from build123d import *

# Parameters (mm, degrees)
SKETCH1_W           = 33.746
SKETCH1_H           = 13.93
SKETCH1_W_2         = 32.946
SKETCH1_H_2         = 13.13
BOSS_EXTRUDE1_DEPTH = 11.37
CUT_EXTRUDE1_DEPTH  = 25.658060122
BOSS_EXTRUDE2_DEPTH = 5
BOSS_EXTRUDE3_DEPTH = 5


with BuildPart() as part:
    # Sketch1 → Boss-Extrude1 (new, symmetric)
    with BuildSketch(Plane.XY):
        Rectangle(SKETCH1_W, SKETCH1_H)
        Rectangle(SKETCH1_W_2, SKETCH1_H_2, mode=Mode.SUBTRACT)
    extrude(amount=BOSS_EXTRUDE1_DEPTH, both=True)

    # Sketch3 → Cut-Extrude1 (cut, through all)
    with BuildSketch(Plane(origin=(0, 6.965, 0), x_dir=(1, 0, 0), z_dir=(0, 1, 0))):
        with BuildLine():
            ThreePointArc((0, 11.37), (8.54007907, 10.702927857), (16.873, 8.717892708))
            Line((16.873, 8.717892708), (16.873, 11.37))
            Line((16.873, 11.37), (0, 11.37))
        make_face()
        with BuildLine():
            Line((-16.873, 11.37), (-16.873, 8.717892708))
            ThreePointArc((-16.873, 8.717892708), (-8.54007907, 10.702927857), (0, 11.37))
            Line((0, 11.37), (-16.873, 11.37))
        make_face()
        with BuildLine():
            ThreePointArc((16.873, -11.37), (0, -7.1709728), (-16.873, -11.37))
            Line((-16.873, -11.37), (16.873, -11.37))
        make_face()
    extrude(amount=-CUT_EXTRUDE1_DEPTH, mode=Mode.SUBTRACT)

    # Sketch4 → Boss-Extrude2 (add)
    with BuildSketch(Plane(origin=(0, 6.965, 0), x_dir=(1, 0, 0), z_dir=(0, 1, 0))):
        with BuildLine():
            Line((-16.873, -11.37), (-16.873, -10.37))
            ThreePointArc((-16.873, -10.37), (0, -6.1709728), (16.873, -10.37))
            Line((16.873, -10.37), (16.873, -11.37))
            ThreePointArc((16.873, -11.37), (0, -7.1709728), (-16.873, -11.37))
        make_face()
        with BuildLine():
            Line((-16.873, 8.717892708), (-16.873, 7.717892708))
            ThreePointArc((-16.873, 7.717892708), (0, 10.37), (16.873, 7.717892708))
            Line((16.873, 7.717892708), (16.873, 8.717892708))
            ThreePointArc((16.873, 8.717892708), (0, 11.37), (-16.873, 8.717892708))
        make_face()
    extrude(amount=BOSS_EXTRUDE2_DEPTH)

    # Sketch5 → Boss-Extrude3 (add)
    with BuildSketch(Plane.XZ.offset(6.965)):
        with BuildLine():
            Line((-16.873, 11.37), (-16.873, 10.37))
            ThreePointArc((-16.873, 10.37), (0, 6.1709728), (16.873, 10.37))
            Line((16.873, 10.37), (16.873, 11.37))
            ThreePointArc((16.873, 11.37), (0, 7.1709728), (-16.873, 11.37))
        make_face()
        with BuildLine():
            Line((-16.873, -8.717892708), (-16.873, -7.717892708))
            ThreePointArc((-16.873, -7.717892708), (0, -10.37), (16.873, -7.717892708))
            Line((16.873, -7.717892708), (16.873, -8.717892708))
            ThreePointArc((16.873, -8.717892708), (0, -11.37), (-16.873, -8.717892708))
        make_face()
    extrude(amount=BOSS_EXTRUDE3_DEPTH)


solid = part.part
Read the model definition and answer for the solid it produces. Units are mm, in the model's axes. A direction names the side the tool comes from. Coordinates: 2 decimals unless noted, no trailing zeros. Write each loop counter-clockwise with the first axis right and the second up, starting at its lowest first coordinate (ties: lowest second). Pieces come first, ordered by that corner, then holes. Notation, with made-up numbers: (50.5, 15) - (84.5, 15) arc R19 cw to (84.5, 49) - close; hole circle Ø1 at (-21, 45.25). An arc over 180 degrees is marked (long way). One line per question, with ' | ' between items.
Q1. Consider L1, parallel to Y at x = 9, z = 4 (3 decimals); L2, parallel to X at y = -2.5, z = -1; L3, parallel to Y at x = 6, z = 7.5 (3 decimals). Determine where each line is inside the solid, lowest interval first. Write a range as [from, to].
Result set:
L1: [-6.965, -6.565], [6.565, 6.965] | L2: [-16.87, -16.47], [16.47, 16.87] | L3: [-11.965, -6.565], [6.565, 11.965]
Q2. Each of these flat-tipped pins is pushed along its axis until it touches: P1, Ø1, axis at x = 7, y = -7, coming from the +Z side; P2, Ø10, axis at x = -3, z = -2, coming from the +Y side (3 decimals); P3, Ø2, axis at x = -10, z = 3, coming from the -Y side (3 decimals). Where does it stop, or does it pass through?
Result set:
P1: z = 7.96 | P2: y = 6.965 | P3: y = -6.965
Q3. Determine the mould class of faces 5 (the flat face through (0, 11.965, 7)), 6 (the flat face through (16.473, 0, 1)), 7 (the cylindrical face through (-0.25, -9.43, 6.17)) for opening direction X: +X half, -X half, draft (parallel to the pull), parting line (faces both ways), or undercut.
Result set:
face 5: draft | face 6: undercut | face 7: parting line
Q4. Find section B-B, the plane x = 1. Write down the section's boundary in (y, z) (3 decimals).
Result set:
outline: (-11.965, -11.361) - (-6.565, -11.361) - (-6.565, 7.185) - (-11.965, 7.185) - (-11.965, 6.185) - (-6.965, 6.185) - (-6.965, -10.361) - (-11.965, -10.361) - close; (6.565, -11.361) - (11.965, -11.361) - (11.965, -10.361) - (6.965, -10.361) - (6.965, 6.185) - (11.965, 6.185) - (11.965, 7.185) - (6.565, 7.185) - close
Q5. For faces 1 (the cylindrical face through (-0.25, 9.43, 6.17)), 2 (the flat face through (0, 6.565, 0)), 3 (the flat face through (-16.873, 0, 1)), 4 (the cylindrical face through (-0.24, -9.43, -10.37)), determine the directions among +Z, -Z, +X, -X, +Y, -Y from which every point of the face is accessible in a straight line to the end or side of a thin tool.
Result set:
face 1: +Y | face 2: +Z, -Z | face 3: +Z, -Z, -X, +Y, -Y | face 4: -Y
Q6. Find section D-D, the plane y = -9.5. Write down the section's boundary in (x, z), plus the area to 3 significant figures.
Result set:
outline: (-16.87, -8.72) arc R55 ccw to (16.87, -8.72) - (16.87, -7.72) arc R55 cw to (-16.87, -7.72) - close; (-16.87, 10.37) arc R36 ccw to (16.87, 10.37) - (16.87, 11.37) arc R36 cw to (-16.87, 11.37) - close | area: 67.5 mm^2
Q7. Find section C-C, the plane z = 5. Write down the section's boundary in (x, y) (3 decimals), plus the area to 3 significant figures.
Result set:
outline: (-16.873, -6.965) - (16.873, -6.965) - (16.873, 6.965) - (-16.873, 6.965) - close; hole (-16.473, -6.565) - (16.473, -6.565) - (16.473, 6.565) - (-16.473, 6.565) - close | area: 37.5 mm^2
Q8. Find section A-A, the plane y = -6. Write down the section's boundary in (x, z), plus the area to 3 significant figures.
Result set:
outline: (-16.87, -8.72) arc R55 ccw to (-16.47, -8.85) - (-16.47, 11.16) arc R36 cw to (-16.87, 11.37) - close; (16.47, -8.85) arc R55 ccw to (16.87, -8.72) - (16.87, 11.37) arc R36 cw to (16.47, 11.16) - close | area: 16.0 mm^2
